Autodesk Inventor part; units mm, degrees
ref_plane "YZ Plane" through (0, 0, 0) normal (1, 0, 0) x (0, 1, 0)
ref_plane "XZ Plane" through (0, 0, 0) normal (0, 1, 0) x (-1, 0, 0)
ref_plane "XY Plane" through (0, 0, 0) normal (0, 0, 1) x (1, 0, 0)
sketch "스케치1" plane through (0, 0, 0) normal (0, 0, 1) x (1, 0, 0)
  line L0 (-25.5, 15) -> (25.5, 15)
  line L1 (25.5, 15) -> (25.5, -15)
  line L2 (25.5, -15) -> (-25.5, -15)
  line L3 (-25.5, -15) -> (-25.5, 15)
  line L4 (-25.5, 15) -> (25.5, -15) construction
  line L5 (25.5, 15) -> (-25.5, -15) construction
  line L6 (-2, -12) -> (23, -12) construction
  line L7 (23, -12) -> (23, 12) construction
  line L8 (23, 12) -> (-2, 12) construction
  line L9 (-2, 12) -> (-2, -12) construction
  line L10 (-2, -12) -> (23, 12) construction
  line L11 (23, -12) -> (-2, 12) construction
  circle A0 centre (-2, 12) radius 1
  line L12 (10.5, 0) -> (13.8415, 0)
  line L13 (10.5, 0) -> (10.5, -2.9401)
  circle A1 centre (23, 12) radius 1
  circle A2 centre (-2, -12) radius 1
  circle A3 centre (23, -12) radius 1
  point P0 (0, 0)
  dimension "d0" = 51
  dimension "d1" = 30
  dimension "d2" = 2
  dimension "d3" = 15
  dimension "d4" = 24
  dimension "d5" = 25
extrude "돌출1" add sketch "스케치1" along normal mid plane 6
sketch "스케치4" plane through (25.5, -15, -3) normal (1, 0, 0) x (0, 0, -1)
  line L0 (-6, -3) -> (0, -3)
  line L1 (0, -3) -> (0, 33)
  line L2 (0, 33) -> (-6, 33)
  line L3 (-6, 33) -> (-6, -3)
  line L4 (-6, -3) -> (0, 33) construction
  line L5 (0, -3) -> (-6, 33) construction
  line L6 (-6, 33) -> (-3, 30)
  line L7 (-3, 30) -> (0, 33)
  line L8 (0.1414, 32.8586) -> (-3, 29.7172)
  line L9 (-3, 29.7172) -> (-6, 32.7172)
  line L10 (-3, 15) -> (-1.4715, 15)
  line L11 (0.1414, -2.8586) -> (-3, 0.2828)
  line L12 (-3, 0.2828) -> (-6, -2.7172)
  line L13 (0, 30) -> (-6, 30)
  line L14 (-6, 0) -> (-6, 30)
  line L15 (0, 0) -> (-6, 0)
  line L16 (0, 30) -> (0, 0)
  point P0 (-6, 0)
  point P1 (0, -2.7172)
  point P2 (-6, 30)
  point P3 (0, 32.7172)
  point P4 (-5, 32.7172)
  point P5 (-2.7172, 0)
  point P6 (-3.2828, 0)
  point P7 (-3.2828, 30)
  point P8 (-2.7172, 30)
  dimension "d25" = 36
  dimension "d27" = 90
  dimension "d28" = 0.2
extrude "돌출3" add sketch "스케치4" against normal up to surface (51 mm away) contours L3 L15 L12 | L11 L15 L1 | L3 L9 L13 | L13 L8 L1
sketch "스케치6" plane through (25.5, -17.7172, 3) normal (1, 0, 0) x (0, 0, -1)
  circle A0 centre (3, 37.7172) radius 3
  circle A1 centre (3, 37.7172) radius 1.25
  line L0 (3, 17.7172) -> (21.0559, 17.7172)
  circle A2 centre (3, -2.2828) radius 3
  circle A3 centre (3, -2.2828) radius 1.25
  line L1 (0, 35.4343) -> (0, 0)
  line L2 (0, 35.4343) -> (0, 37.7172)
  line L3 (6, 0) -> (6, 35.4343)
  line L4 (6, 37.7172) -> (6, 35.4343)
  line L5 (0, -2.2828) -> (0, 0)
  line L6 (6, -2.2828) -> (6, 0)
  line L7 (3.2828, 32.7172) -> (2.7172, 32.7172)
  line L8 (2.7172, 32.7172) -> (0, 35.4343)
  line L9 (0, 35.4343) -> (0, 0)
  line L10 (0, 0) -> (2.7172, 2.7172)
  line L11 (3.2828, 2.7172) -> (2.7172, 2.7172)
  line L12 (3.2828, 2.7172) -> (6, 0)
  line L13 (6, 0) -> (6, 35.4343)
  line L14 (6, 35.4343) -> (3.2828, 32.7172)
  dimension "d36" = 6
  dimension "d37" = 2.5
  dimension "d38" = 40
extrude "돌출5" add sketch "스케치6" against normal blind 5 contours A0 | L4 L14 L7 L8 L2 A0 | L10 L11 L12 L6 A2 L5 | A2
sketch "스케치7" plane through (0, 0, 3) normal (0, 0, 1) x (1, 0, 0)
  circle A0 centre (-2, 12) radius 1
  circle A1 centre (-2, 12) radius 2
  circle A2 centre (23, 12) radius 1
  circle A3 centre (23, 12) radius 2
  circle A4 centre (-2, -12) radius 1
  circle A5 centre (-2, -12) radius 2
  circle A6 centre (23, -12) radius 1
  circle A7 centre (23, -12) radius 2
  point P0 (0, 0)
  dimension "d41" = 4
  dimension "d42" = 4
  dimension "d43" = 4
  dimension "d44" = 4
extrude "돌출6" add sketch "스케치7" along normal blind 2
fillet "모깎기1" radius 2 4 edges at (-4, 12, 3) (21, 12, 3) (-4, -12, 3) (21, -12, 3)
properties part number "카메라 홀더"
Input: part model. Units: mm. Frame: model coordinates. A direction names the side the tool comes from. Give positions to 0.01 mm unless a question says otherwise; leave off trailing zeros. Loops run counter-clockwise (first coordinate to the right, second up) from the corner with the lowest first, then second, coordinate; pieces in that order, holes last. Notation, with made-up numbers: M -39.75,-37 L -0.75,-37 A28 cw -0.75,-9 Z; hole C -1,8.5 d1. An arc over 180 degrees is marked long. Use one line per item in the form item = value.
1. First-contact query: pin 1 (0.5 mm diameter, centred on x = 0, z = 0, fed in from +Y); pin 2 (2 mm diameter, centred on y = 20, z = 0, fed in from +X); pin 3 (1.8 mm diameter, centred on y = 18, z = 1, fed in from -X); pin 4 (1.5 mm diameter, centred on x = 4.5, z = 3, fed in from +Y). Flat tips, straight axial feed; report the tip coordinate or a pass-through.
Numbers:
pin_1 = 15
pin_2 = through
pin_3 = 20.5
pin_4 = 17.72
2. Section query B-B, the plane x = 23. Return the cut outline in (y, z).
Numbers:
outline = M -20,-3 L -13,-3 L -13,5 L -14,5 A2 cw -16,3 L -20,3 A3 ccw Z; M -11,-3 L 11,-3 L 11,5 L 10,5 A2 cw 8,3 L -8,3 A2 cw -10,5 L -11,5 Z; M 13,-3 L 20,-3 A3 ccw 20,3 L 16,3 A2 cw 14,5 L 13,5 Z; hole C -20,0 d2.5; hole C 20,0 d2.5
3. Line query: L1, parallel to Y at x = 21.85, z = 0; L2, parallel to X at y = -12.5, z = -0.75; L3, parallel to Y at x = 23, z = 2.25. Output: solid intervals per line, ascending.
Numbers:
L1 = -23 to -21.25, -18.75 to 18.75, 21.25 to 23
L2 = -25.5 to -2.87, -1.13 to 22.13, 23.87 to 25.5
L3 = -21.98 to -13, -11 to 11, 13 to 21.98
4. Section query D-D, the plane x = -2. Return the cut outline in (y, z), and give its area (3 significant figures).
Numbers:
outline = M -17.72,-3 L -13,-3 L -13,5 L -14,5 A2 cw -16,3 L -17.72,3 L -15,0.28 L -15,-0.28 Z; M -11,-3 L 11,-3 L 11,5 L 10,5 A2 cw 8,3 L -8,3 A2 cw -10,5 L -11,5 Z; M 13,-3 L 17.72,-3 L 15,-0.28 L 15,0.28 L 17.72,3 L 16,3 A2 cw 14,5 L 13,5 Z
area = 182 mm²
5. Section query A-A, the plane y = -12. Return the cut outline in (x, z).
Numbers:
outline = M -25.5,-3 L -3,-3 L -3,5 L -4,5 A2 cw -6,3 L -25.5,3 Z; M -1,-3 L 22,-3 L 22,5 L 21,5 A2 cw 19,3 L 2,3 A2 cw 0,5 L -1,5 Z; M 24,-3 L 25.5,-3 L 25.5,3.68 A2 cw 25,5 L 24,5 Z
6. Section query C-C, the plane z = 2. Return the cut outline in (x, y).
Numbers:
outline = M -25.5,-16.72 L 20.5,-16.72 L 20.5,-22.24 L 25.5,-22.24 L 25.5,22.24 L 20.5,22.24 L 20.5,16.72 L -25.5,16.72 Z; hole C -2,-12 d2; hole C -2,12 d2; hole C 23,-12 d2; hole C 23,12 d2
7. Reachability of faces 1 (the face through (-2.18, -16.38, -1.66)), 2 (the face through (0, 4, 3)), 3 (the face through (-2.18, 16.34, 1.62)) from +Z, -Z, +X, -X, +Y, -Y: full face, straight path, thin tool, end or side. Return the list, or none.
Numbers:
face_1 = -X, -Y
face_2 = +Z
face_3 = -X, +Y
8. Pull-direction query (X, two-part tool) for faces 4 (the face through (-2.18, 16.38, -1.66)), 5 (the face through (-2.737, 11.324, 0.944)), 6 (the face through (20.5, 18, 0)); classes: released by +X, released by -X, zero draft, split by the parting line, or undercut.
Numbers:
face_4 = zero draft
face_5 = undercut
face_6 = released by -X
